Autodesk Inventor part; units mm, degrees
ref_plane "YZ Plane" through (0, 0, 0) normal (1, 0, 0) x (0, 1, 0)
ref_plane "XZ Plane" through (0, 0, 0) normal (0, 1, 0) x (-1, 0, 0)
ref_plane "XY Plane" through (0, 0, 0) normal (0, 0, 1) x (1, 0, 0)
sketch "Sketch1" plane through (0, 0, 0) normal (0, 1, 0) x (-1, 0, 0)
  line L0 (0, 0) -> (80, 0)
  line L1 (80, 0) -> (80, -80)
  line L2 (80, -80) -> (0, -80)
  line L3 (0, -80) -> (0, 0)
  circle A0 centre (40, -40) radius 15
  line L4 (20, 0) -> (0, -20)
  point P0 (80, -40)
  point P1 (40, -80)
  dimension "d0" = 80
  dimension "d1" = 80
  dimension "d3" = 30
  dimension "d4" = 20
  dimension "d5" = 20
extrude "Extrusion1" add sketch "Sketch1" along normal blind 10 contours L0 L1 L2 L3 L4
sketch "Sketch2" plane through (0, 10, 0) normal (0, 1, 0) x (1, 0, 0)
  line L0 (0, 80) -> (-80, 80)
  line L1 (0, 20) -> (0, 80)
  line L2 (-80, 80) -> (0, 80)
  line L3 (0, 80) -> (0, 70)
  line L4 (0, 70) -> (-80, 70)
  line L5 (-80, 70) -> (-80, 80)
  line L6 (-80, 80) -> (-80, 0)
  line L7 (-80, 0) -> (-70, 0)
  line L8 (-70, 0) -> (-70, 80)
  line L9 (-70, 80) -> (-80, 80)
  line L10 (-80, 80) -> (-80, 0)
  point P0 (0, 0)
  point P1 (-70, 70)
  dimension "d8" = 10
  dimension "d9" = 10
extrude "Extrusion2" add sketch "Sketch2" along normal blind 40
fillet "Fillet1" radius 5 1 edges at (-70, 30, -70)
fillet "Fillet2" radius 15 1 edges at (-80, 25, -80)
sketch "Sketch3" plane through (0, 10, -70) normal (0, 0, 1) x (1, 0, 0)
  circle A0 centre (-32.5, 20) radius 7.5
  line L0 (0, 0) -> (0, 40)
  line L1 (-65, 40) -> (0, 40)
  line L2 (-80, -10) -> (-80, 40)
  point P0 (0, -10)
  point P1 (0, 20)
  point P2 (-32.5, 40)
  point P3 (-32.5, 40)
  point P4 (0, 20)
  point P5 (0, 20)
  point P6 (0, 20)
  dimension "d14" = 15
  dimension "d15" = 80
extrude "Extrusion3" cut sketch "Sketch3" against normal blind 40
sketch "Sketch4" plane through (-70, 10, 0) normal (1, 0, 0) x (0, 0, -1)
  circle A0 centre (32.4993, 20) radius 7.5
  line L0 (65, 40) -> (65, 0)
  line L1 (0, 0) -> (0, 40)
  point P0 (0, -10)
  point P1 (0, 20)
  dimension "d18" = 15
  dimension "d19" = 65
  dimension "d20" = 32.4993
extrude "Extrusion4" cut sketch "Sketch4" against normal blind 40
fillet "Fillet3" radius 1 14 edges at (-32.5, 50, -70) (-70, 50, -32.5) (-70, 30, 0) (-68.5355, 10, -68.5355) (-32.5, 10, -70) (-70, 10, -32.5) (-45, 10, 0) (-10, 10, -10) (0, 10, -45) (0, 30, -70) (-70, 30, -24.9993) (-40, 30, -70) (-40, 30, -80) (-80, 30, -24.9993)
properties part number "Tutorial Pt.1" material "Stainless Steel"
Geometry check sheet. Reference: the model listing, model coordinates, mm. A direction names the side the tool comes from. Round coordinates to 2 decimals unless told otherwise and drop trailing zeros. Loops run counter-clockwise (first coordinate to the right, second up) from the corner with the lowest first, then second, coordinate; pieces in that order, holes last. Notation, with made-up numbers: (63, 1.5) - (74, 1.5) arc R17 ccw to (74, 14.5) - close; hole circle Ø2 at (-21.5, 89). An arc over 180 degrees is marked (long way). Write item = value, one per line. Start each with the question number.
1. Depth check by flat-ended pin: pin 1 (17 mm diameter, centred on x = -32.5, y = 30, fed in from +Z); pin 2 (8 mm diameter, centred on x = -38.5, z = -61.5, fed in from -Y); pin 3 (2 mm diameter, centred on x = -33, y = 11.5, fed in from +Z); pin 4 (1.5 mm diameter, centred on y = 36.5, z = -19.5, fed in from +X). Enter the tip coordinate at first touch or a pass-through.
2. Section check A-A on y = 30. Enter the section's corners in (x, z).
3. Section check B-B on z = -45. Enter the section's corners in (x, y), then the cut area to 3 significant figures.
4. Mould release check, pull along Y, two halves, no side actions. Record for faces 3 (the face through (-27, 10, -27)), 4 (the face through (-10, 4, -10)), 5 (the face through (-34.13, 22.68, -74.94)): released by +Y, released by -Y, zero draft, split by the parting line, or undercut.
5. Set-up check for faces 1 (the face through (-68, 30, -69)), 2 (the face through (-75.72, 24.65, -75.49)): record each of +Z, -Z, +X, -X, +Y, -Y from which the full face is reachable in a straight line by a thin tool's end or side.
6. Thickness scan on line 1 (Y direction, x = -32, z = -73); line 2 (Z direction, x = -40, y = 3); line 3 (Y direction, x = -12, z = -51). Record the ranges inside material, lowest first.
7. Section check C-C on x = -32.5. Enter the section's corners in (y, z).
8. Section check D-D on z = -22.5. Enter the section's corners in (x, y), then the cut area to 3 significant figures.
Working result:
q1.pin_1 = -70
q1.pin_2 = 0
q1.pin_3 = -69.87
q1.pin_4 = -70
q2.outline = (-80, -65) arc R15 ccw to (-65, -80) - (-41, -80) arc R1 ccw to (-40, -79) - (-40, -71) arc R1 ccw to (-41, -70) - (-65, -70) arc R5 cw to (-70, -65) - (-70, -41) arc R1 ccw to (-71, -40) - (-79, -40) arc R1 ccw to (-80, -41) - close; (-80, -24) arc R1 ccw to (-79, -25) - (-71, -25) arc R1 ccw to (-70, -24) - (-70, -1) arc R1 ccw to (-71, 0) - (-80, 0) - close; (-25, -79) arc R1 ccw to (-24, -80) - (0, -80) - (0, -71) arc R1 ccw to (-1, -70) - (-24, -70) arc R1 ccw to (-25, -71) - close
q3.outline = (-80, 0) - (-54.14, 0) - (-54.14, 10) - (-69, 10) arc R1 cw to (-70, 11) - (-70, 49) arc R1 ccw to (-71, 50) - (-80, 50) - close; (-25.86, 0) - (0, 0) - (0, 9) arc R1 ccw to (-1, 10) - (-25.86, 10) - close
q3.area = 917 mm^2
q4.face_3 = released by +Y
q4.face_4 = zero draft
q4.face_5 = undercut
q5.face_1 = +Z, +X, +Y
q5.face_2 = -Z, -X, +Y, -Y
q6.line_1 = 0 to 22.52, 37.48 to 50
q6.line_2 = -80 to -55, -25 to 0
q6.line_3 = 0 to 10
q7.outline = (0, -80) - (21.5, -80) arc R1 ccw to (22.5, -79) - (22.5, -71) arc R1 ccw to (21.5, -70) - (11, -70) arc R1 cw to (10, -69) - (10, -52.99) - (0, -52.99) - close; (0, -27.01) - (10, -27.01) - (10, -1) arc R1 ccw to (9, 0) - (0, 0) - close; (37.5, -79) arc R1 ccw to (38.5, -80) - (50, -80) - (50, -71) arc R1 ccw to (49, -70) - (38.5, -70) arc R1 ccw to (37.5, -71) - close
q8.outline = (-80, 0) - (0, 0) - (0, 9) arc R1 ccw to (-1, 10) - (-69, 10) arc R1 cw to (-70, 11) - (-70, 49) arc R1 ccw to (-71, 50) - (-80, 50) - close
q8.area = 1,200 mm^2
